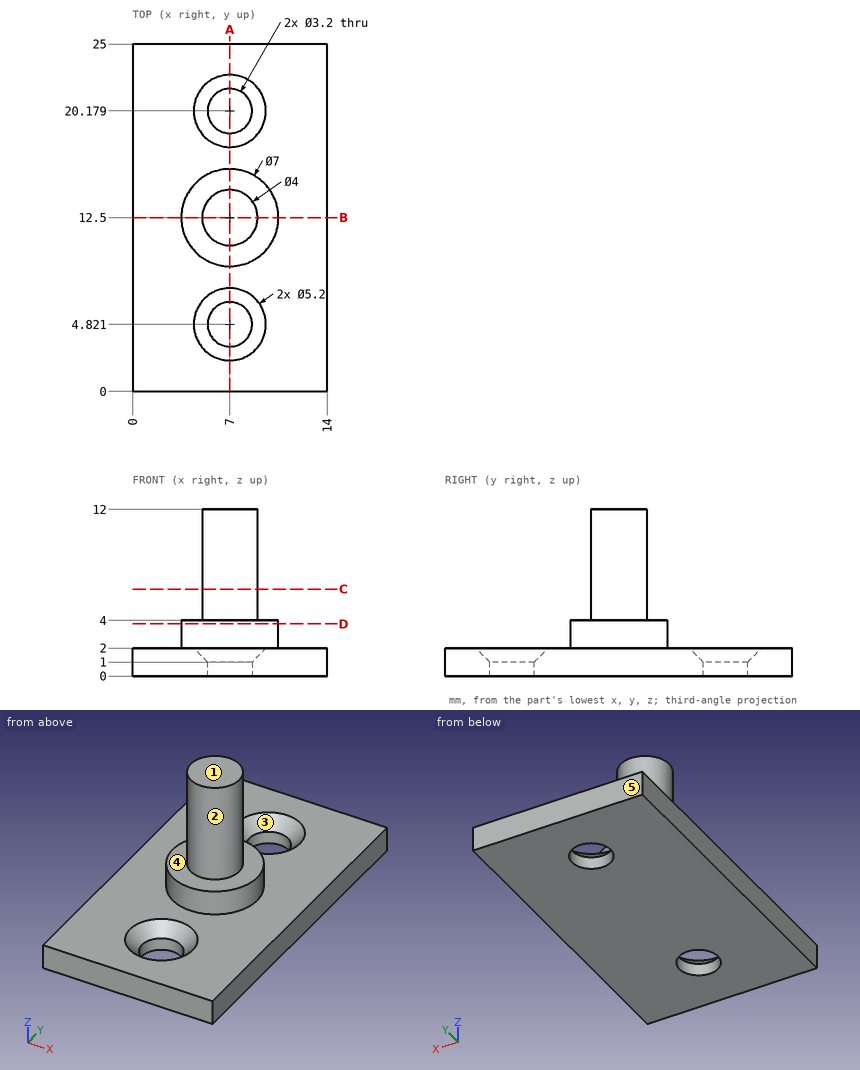
Source: three-view drawing plus pictorial views. Frame: mm from the lowest corner of the part. A direction names the side the tool comes from. Give positions to 0.01 mm unless a question says otherwise; leave off trailing zeros. Loops run counter-clockwise (first coordinate to the right, second up) from the corner with the lowest first, then second, coordinate; pieces in that order, holes last.
1) Reachability of the marked faces 4 and 5 from +Z, -Z, +X, -X, +Y, -Y: full face, straight path, thin tool, end or side. Return the list, or none.
A:
face 4: +Z
face 5: +Z, -Z, +X, -X, +Y
2) Section query C-C on z = 6.25. Return the cut outline in (x, y).
A:
outline: circle Ø4 at (7, 12.5)
3) Line query: L1, parallel to Y at x = 7, z = 0.55; L2, parallel to Z at x = 4.5, y = 3.75; L3, parallel to Z at x = 10, y = 13. Output: solid intervals per line, ascending.
A:
L1: y = 0 to 3.22, 6.42 to 18.58, 21.78 to 25
L2: z = 0 to 2
L3: z = 0 to 4
4) Contact query for flat-ended pins moving along their axis: pin 1 (3 mm diameter, centred on x = 7, y = 20.18, fed in from +Z); pin 2 (6 mm diameter, centred on x = 5.5, z = 9, fed in from -Y); pin 3 (5 mm diameter, centred on x = 7, y = 6, fed in from +Z); pin 4 (5 mm diameter, centred on x = 3, z = 5.5, fed in from +Y). Output: stop coordinate, or through.
A:
pin 1: passes through
pin 2: stops at y = 10.5
pin 3: stops at z = 2
pin 4: stops at y = 15.37
5) Section query A-A on x = 7. Return the cut outline in (y, z).
A:
outline: (0, 0) - (3.22, 0) - (3.22, 1) - (2.22, 2) - (0, 2) - close; (6.42, 0) - (18.58, 0) - (18.58, 1) - (17.58, 2) - (16, 2) - (16, 4) - (14.5, 4) - (14.5, 12) - (10.5, 12) - (10.5, 4) - (9, 4) - (9, 2) - (7.42, 2) - (6.42, 1) - close; (21.78, 0) - (25, 0) - (25, 2) - (22.78, 2) - (21.78, 1) - close
6) Mould query, pull axis Y, two halves, no side actions, for the marked faces 1, 2 and 3. Classes: released by +Y, released by -Y, zero draft, split by the parting line, or undercut.
A:
face 1: zero draft
face 2: split by the parting line
face 3: undercut
7) Section query D-D on z = 3.75. Return the cut outline in (x, y).
A:
outline: circle Ø7 at (7, 12.5)
8) Section query B-B on y = 12.5. Return the cut outline in (x, z), and give its area (3 significant figures).
A:
outline: (0, 0) - (14, 0) - (14, 2) - (10.5, 2) - (10.5, 4) - (9, 4) - (9, 12) - (5, 12) - (5, 4) - (3.5, 4) - (3.5, 2) - (0, 2) - close
area: 74.0 mm2
